```python
from build123d import *

# Parameters (mm, degrees)
F0_W           = 90
F0_H           = 60
F1_DEPTH       = 18
F3_D           = 6
F3_CBORE_D     = 10
F3_CBORE_DEPTH = 5
F7_DEPTH       = 30


with BuildPart() as f1:
    # F0 (on Front) → F1 (new body)
    with BuildSketch(Plane.XZ):
        with Locations((0, 30)):
            Rectangle(F0_W, F0_H)
    extrude(amount=F1_DEPTH)

    # F3 (through all)
    with Locations(Plane.XZ.offset(18)):
        with Locations((-27.5, 35), (-17.5, 25), (17.5, 25), (27.5, 35)):
            CounterBoreHole(F3_D / 2, F3_CBORE_D / 2, F3_CBORE_DEPTH)

    # F6 (on offset) → F7 (cut, through all)
    with BuildSketch(Plane(origin=(-15, 0, 0), x_dir=(0, -1, 0), z_dir=(-1, 0, 0))):
        Polygon((15.5, 0), (18, 0), (18, 5), align=None)
    extrude(amount=-F7_DEPTH, mode=Mode.SUBTRACT)


solid = f1.part
```
Geometry check sheet. Reference: the model listing, model coordinates, mm. A direction names the side the tool comes from. Round coordinates to 2 decimals unless told otherwise and drop trailing zeros. Order: outer loops, then holes, each group sorted by start corner. A loop starts at its lowest first (then second) coordinate and runs counter-clockwise, first axis right, second up. Notation, with made-up numbers: (49, 82) - (56, 82) arc R31 ccw to (56, 118) - close; hole circle Ø3 at (-8.75, 81.25). An arc over 180 degrees is marked (long way). Use a Markdown table: item, result. Add a question column.
(1) Sectioned sample at D-D, the plane x = -28. Enter the section's corners in (y, z), and give its area (3 significant figures).
(2) Sectioned sample at C-C, the plane y = -2.5. Enter the section's corners in (x, z).
(3) Depth check by flat-ended pin: pin 1 (5 mm diameter, centred on x = -30, z = 46, fed in from +Y); pin 2 (7 mm diameter, centred on x = -27.5, z = 35, fed in from -Y); pin 3 (3 mm diameter, centred on x = 27.5, z = 35, fed in from -Y). Enter the tip coordinate at first touch or a pass-through.
(4) Tool access check on faces 4 (the flat face through (0, -17, 3)), 5 (the cylindrical face through (-31.185, -15.535, 38.379)), 6 (the cylindrical face through (29.71, -6.41, 37.03)). Record the directions out of +Z, -Z, +X, -X, +Y, -Y that give a thin tool (end or side, any length) a straight path to the whole face; none if there is none.
(5) Release check for a two-part mould opening along X. For faces 1 (the flat face through (-45, -9, 30)), 2 (the flat face through (-1, -9, 60)), 3 (the flat face through (-15, -13, 23)) record: pulls with the +X half, pulls with the -X half, needs draft (parallel to the pull), parting line crosses it, or undercut.
(6) Sectioned sample at A-A, the plane z = 25. Enter the section's corners in (x, y).
(7) Sectioned sample at B-B, the plane x = 27.5. Enter the section's corners in (y, z), and give its area (3 significant figures).
(8) Material ranges on line 1 along Z through (x, y) = (27.5, -15); line 2 along Z through (x, y) = (17.5, -15.5); line 3 along X through (y, z) = (-12.75, 26), recorded low to high. Write a range as [from, to].
Answers below:
| question | item | result |
|---|---|---|
| 1 | outline | (-18, 0) - (0, 0) - (0, 32.04) - (-13, 32.04) - (-13, 30.03) - (-18, 30.03) - close; (-18, 39.97) - (-13, 39.97) - (-13, 37.96) - (0, 37.96) - (0, 60) - (-18, 60) - close |
| 1 | area | 953 mm² |
| 2 | outline | (-45, 0) - (45, 0) - (45, 60) - (-45, 60) - close; hole circle Ø6 at (-27.5, 35); hole circle Ø6 at (-17.5, 25); hole circle Ø6 at (17.5, 25); hole circle Ø6 at (27.5, 35) |
| 3 | pin 1 | y = 0 |
| 3 | pin 2 | y = -13 |
| 3 | pin 3 | through |
| 4 | face 4 | -Z, -Y |
| 4 | face 5 | -Y |
| 4 | face 6 | +Y, -Y |
| 5 | face 1 | pulls with the -X half |
| 5 | face 2 | needs draft |
| 5 | face 3 | undercut |
| 6 | outline | (-45, -18) - (-22.5, -18) - (-22.5, -13) - (-20.5, -13) - (-20.5, 0) - (-45, 0) - close; (-14.5, -13) - (-12.5, -13) - (-12.5, -18) - (12.5, -18) - (12.5, -13) - (14.5, -13) - (14.5, 0) - (-14.5, 0) - close; (20.5, -13) - (22.5, -13) - (22.5, -18) - (45, -18) - (45, 0) - (20.5, 0) - close |
| 7 | outline | (-18, 0) - (0, 0) - (0, 32) - (-13, 32) - (-13, 30) - (-18, 30) - close; (-18, 40) - (-13, 40) - (-13, 38) - (0, 38) - (0, 60) - (-18, 60) - close |
| 7 | area | 952 mm² |
| 8 | line 1 | [0, 30], [40, 60] |
| 8 | line 2 | [0, 20], [30, 60] |
| 8 | line 3 | [-45, -20.33], [-14.67, 14.67], [20.33, 45] |
